The model under review builds one solid part; all positions refer to its coordinate system, in mm. Coordinates: 2 decimals unless noted, no trailing zeros. Order: outer loops, then holes, each group sorted by start corner. A loop starts at its lowest first (then second) coordinate and runs counter-clockwise, first axis right, second up. Notation, with made-up numbers: (-21.5, 61.25) -> (29.5, 61.25) arc R21 cw to (29.5, 99.25) -> close; hole circle Ø9 at (52, -3). An arc over 180 degrees is marked (long way). Use one line per item in the form item = value. Start each with the question number.
(1) Take a section at A-A (y = -8.5). State the section outline as (x, z) points, then the cut area to 3 significant figures.
(2) Insertion check: pin 1 Ø6 at (x, z) = (95, 70) entering from +Y; pin 2 Ø16 at (x, z) = (95, -70) entering from -Y; pin 3 Ø13 at (x, z) = (-95, -70) entering from +Y. Each pin has a flat end and moves straight along its axis. Give the tip position at first contact, or say it passes through.
(3) Wall thickness on line 1 along Z through (x, y) = (95, -14.5); line 2 along Z through (x, y) = (-92, -3.25); line 3 along X through (y, z) = (-18, 72): over which ranges is each line inside the solid? List them lowest first.
```python
from build123d import *

# Parameters (mm, degrees)
F0_W           = 250
F0_H           = 200
F1_DEPTH       = 25
F2_R           = 30
F4_D           = 10
F4_CBORE_D     = 20
F4_CBORE_DEPTH = 5
F5_R           = 2


with BuildPart() as f1:
    # F0 (on Front) → F1 (new body)
    with BuildSketch(Plane.XZ):
        Rectangle(F0_W, F0_H)
    extrude(amount=F1_DEPTH)

    # F2
    f2_edges = [f1.edges().sort_by_distance(p)[0] for p in [
        (-125, -12.5, 100),
        (-125, -12.5, -100),
        (125, -12.5, 100),
        (125, -12.5, -100),
    ]]
    fillet(f2_edges, radius=F2_R)

    # F4 (through all)
    with Locations(Plane.XZ.offset(25)):
        with Locations((-95, 70), (-95, -70), (95, -70), (95, 70)):
            CounterBoreHole(F4_D / 2, F4_CBORE_D / 2, F4_CBORE_DEPTH)

    # F5
    f5_edges = [f1.edges().sort_by_distance(p)[0] for p in [
        (0, 0, -100),
    ]]
    fillet(f5_edges, radius=F5_R)


solid = f1.part
```
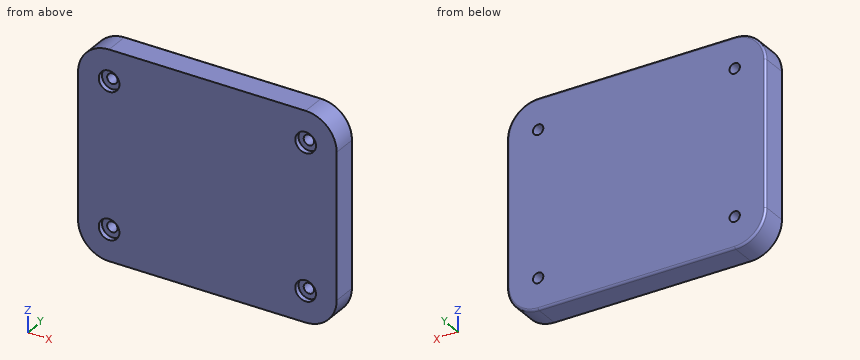
Findings:
q1.outline = (-125, -70) arc R30 ccw to (-95, -100) -> (95, -100) arc R30 ccw to (125, -70) -> (125, 70) arc R30 ccw to (95, 100) -> (-95, 100) arc R30 ccw to (-125, 70) -> close; hole circle Ø10 at (-95, -70); hole circle Ø10 at (-95, 70); hole circle Ø10 at (95, -70); hole circle Ø10 at (95, 70)
q1.area = 48,900 mm²
q2.pin_1 = through
q2.pin_2 = -20
q2.pin_3 = 0
q3.line_1 = -100 to -75, -65 to 65, 75 to 100
q3.line_2 = -100 to -74, -66 to 66, 74 to 100
q3.line_3 = -124.93 to -99.58, -90.42 to 90.42, 99.58 to 124.93
